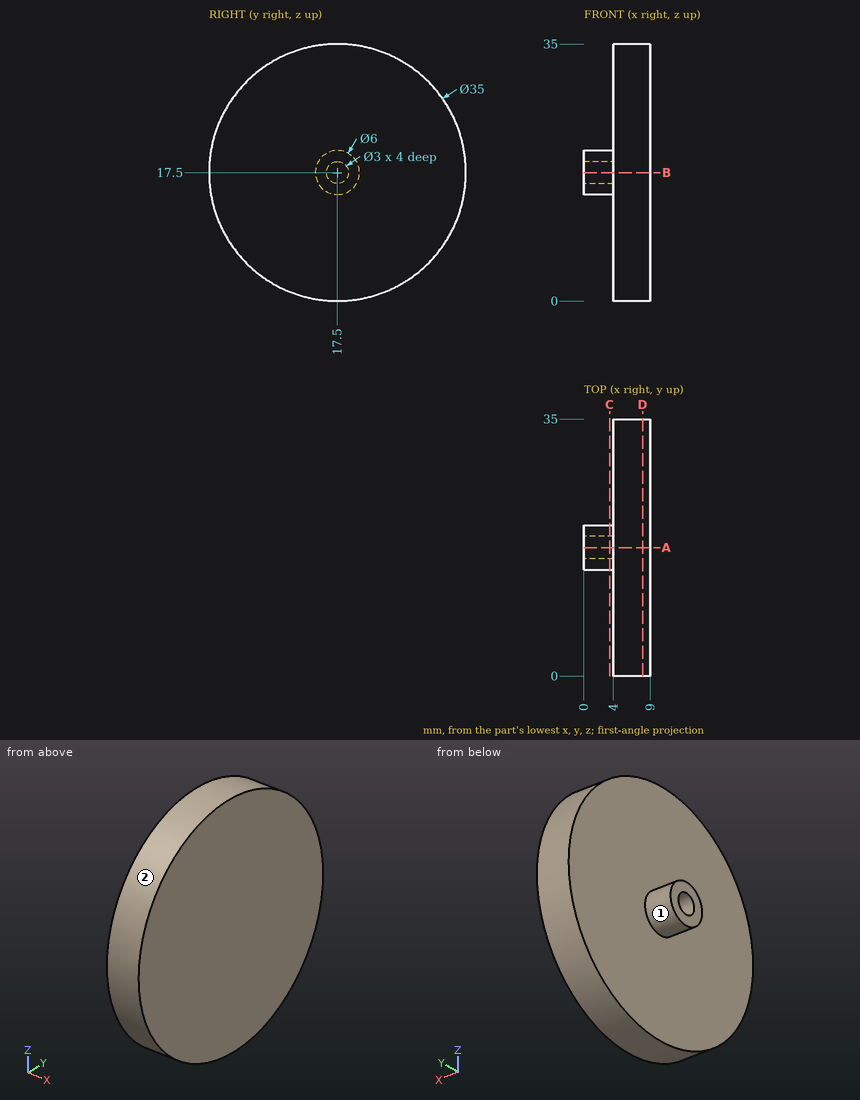
Input: dimensioned drawing with shaded views. Units: mm. Origin: part minimum x, y, z. A direction names the side the tool comes from. Give positions to 0.01 mm unless a question says otherwise; leave off trailing zeros. Write each loop counter-clockwise with the first axis right and the second up, starting at its lowest first coordinate (ties: lowest second). Pieces come first, ordered by that corner, then holes.
1. Section query C-C (x = 3.5). Return the cut outline in (y, z), then the cut area to 3 significant figures.
2. Section query A-A (y = 17.5). Return the cut outline in (x, z).
3. Material intervals for line 1 along Y through (x, z) = (2.6, 17.5); line 2 along X through (y, z) = (17.5, 1); line 3 along Z through (x, y) = (3.75, 18.5), sorted ascending.
4. First-contact query: pin 1 (1.5 mm diameter, centred on x = 3.5, z = 11, fed in from +Y); pin 2 (4 mm diameter, centred on y = 17.5, z = 17.5, fed in from -X); pin 3 (6 mm diameter, centred on y = 26, z = 11.5, fed in from -X); pin 4 (4 mm diameter, centred on x = 5.5, z = 8, fed in from +Y). Flat tips, straight axial feed; report the tip coordinate or a pass-through.
5. Section query D-D (x = 8). Return the cut outline in (y, z).
6. Access query for the marked faces 1 and 2. Directions: +Z, -Z, +X, -X, +Y, -Y. A direction counts if a zero-diameter tool reaches every point of the face in a straight line with its end or side. Return the directions, or none.
Output values:
1. outline: circle Ø6 at (17.5, 17.5); hole circle Ø3 at (17.5, 17.5)
1. area: 21.2 mm2
2. outline: (0, 14.5) - (4, 14.5) - (4, 0) - (9, 0) - (9, 35) - (4, 35) - (4, 20.5) - (0, 20.5) - (0, 19) - (4, 19) - (4, 16) - (0, 16) - close
3. line 1: y = 14.5 to 16, 19 to 20.5
3. line 2: x = 4 to 9
3. line 3: z = 14.67 to 16.38, 18.62 to 20.33
4. pin 1: stops at y = 33.96
4. pin 2: stops at x = 0
4. pin 3: stops at x = 4
4. pin 4: stops at y = 33.31
5. outline: circle Ø35 at (17.5, 17.5)
6. face 1: -X
6. face 2: +X, -X
